from build123d import *

# Parameters (mm, degrees)
ESQUISSE4_R             = 31.794871795
BOSS_EXTRU_1_DEPTH      = 10
ESQUISSE5_R             = 10.8
ESQUISSE5_R_2           = 9
ESQUISSE5_R_3           = 4
BOSS_EXTRU_2_DEPTH      = 10
ESQUISSE6_R             = 4
ENL_V_MAT_EXTRU_2_DEPTH = 5
ESQUISSE8_R             = 4.222540961
ENL_V_MAT_EXTRU_4_DEPTH = 10


with BuildPart() as part:
    # Esquisse4 → Boss.-Extru.1 (new body)
    with BuildSketch(Plane.XY):
        Circle(ESQUISSE4_R)
    extrude(amount=-BOSS_EXTRU_1_DEPTH)

    # Esquisse5 → Boss.-Extru.2 (add)
    # profile 1 of 6: a face of its own
    with BuildSketch(Plane.XY):
        with Locations((15.588457268, -9)):
            Circle(ESQUISSE5_R)
        with Locations((15.588457268, -9)):
            Circle(ESQUISSE5_R_2, mode=Mode.SUBTRACT)
    # profile 2 of 6: a face of its own
    with BuildSketch(Plane.XY):
        with Locations((-15.588457268, -9)):
            Circle(ESQUISSE5_R)
        with Locations((-15.588457268, -9)):
            Circle(ESQUISSE5_R_2, mode=Mode.SUBTRACT)
    # profile 3 of 6: a face of its own
    with BuildSketch(Plane.XY):
        with Locations((0, 18)):
            Circle(ESQUISSE5_R)
        with Locations((0, 18)):
            Circle(ESQUISSE5_R_2, mode=Mode.SUBTRACT)
    # profile 4 of 6: a face of its own
    with BuildSketch(Plane.XY):
        with Locations((21.650635095, 12.5)):
            Circle(ESQUISSE5_R_3)
    # profile 5 of 6: a face of its own
    with BuildSketch(Plane.XY):
        with Locations((-21.650635095, 12.5)):
            Circle(ESQUISSE5_R_3)
    # profile 6 of 6: a face of its own
    with BuildSketch(Plane.XY):
        with Locations((0, -25)):
            Circle(ESQUISSE5_R_3)
    extrude(amount=BOSS_EXTRU_2_DEPTH)

    # Esquisse6 → Enlèv. mat.-Extru.2 (cut)
    with BuildSketch(Plane(origin=(0, 0, -10), x_dir=(-1, 0, 0), z_dir=(0, 0, -1))):
        with Locations((0, 25.641025641)):
            Circle(ESQUISSE6_R)
        with Locations((22.205779584, 12.820512821)):
            Circle(ESQUISSE6_R)
        with Locations((22.205779584, -12.820512821)):
            Circle(ESQUISSE6_R)
        with Locations((0, -25.641025641)):
            Circle(ESQUISSE6_R)
        with Locations((-22.205779584, -12.820512821)):
            Circle(ESQUISSE6_R)
        with Locations((-22.205779584, 12.820512821)):
            Circle(ESQUISSE6_R)
    extrude(amount=-ENL_V_MAT_EXTRU_2_DEPTH, mode=Mode.SUBTRACT)

    # Esquisse8 → Enlèv. mat.-Extru.4 (cut)
    with BuildSketch(Plane(origin=(0, 0, -10), x_dir=(-1, 0, 0), z_dir=(0, 0, -1))):
        Circle(ESQUISSE8_R)
    extrude(amount=-ENL_V_MAT_EXTRU_4_DEPTH, mode=Mode.SUBTRACT)


solid = part.part
Here's how the part is built. I have some questions about the finished solid (model axes, mm). A direction names the side the tool comes from. Coordinates: 2 decimals unless noted, no trailing zeros. Order: outer loops, then holes, each group sorted by start corner. A loop starts at its lowest first (then second) coordinate and runs counter-clockwise, first axis right, second up.
Item 1: If we section it at A-A on x = 0: List the corners of the cut face in (y, z) for me, plus the area to 3 significant figures.
Result sheet:
outline: (-31.79, -10) - (-29.64, -10) - (-29.64, -5) - (-21.64, -5) - (-21.64, -10) - (-4.22, -10) - (-4.22, 0) - (-21, 0) - (-21, 10) - (-29, 10) - (-29, 0) - (-31.79, 0) - close; (4.22, -10) - (21.64, -10) - (21.64, -5) - (29.64, -5) - (29.64, -10) - (31.79, -10) - (31.79, 0) - (28.8, 0) - (28.8, 10) - (27, 10) - (27, 0) - (9, 0) - (9, 10) - (7.2, 10) - (7.2, 0) - (4.22, 0) - close
area: 587 mm2
Item 2: If we mould it in two halves opening along X, with no side actions, what happens to faces 1 (the face through (13, 0, 10)), 2 (the face through (-0.521, -21.034, 4.93)), 3 (the face through (-1.172, 26.923, 4.93))? For each: +X half, -X half, draft (parallel to the pull), parting line (faces both ways), or undercut.
Result sheet:
face 1: draft
face 2: parting line
face 3: undercut
Item 3: If we section it at D-D on y = 23.5: List the corners of the cut face in (x, z) for me.
Result sheet:
outline: (-21.42, -10) - (-3.38, -10) - (-3.38, -5) - (3.38, -5) - (3.38, -10) - (21.42, -10) - (21.42, 0) - (9.29, 0) - (9.29, 10) - (7.12, 10) - (7.12, 0) - (-7.12, 0) - (-7.12, 10) - (-9.29, 10) - (-9.29, 0) - (-21.42, 0) - close
Item 4: For faces 4 (the face through (15, -9, 0)), 5 (the face through (-22, 13, 10)), 6 (the face through (-21.339, -16.725, -7.535)), which set-ups out of +Z, -Z, +X, -X, +Y, -Y let a thin tool reach every point of the face, with its end or its side?
Result sheet:
face 4: +Z
face 5: +Z, +X, -X, +Y, -Y
face 6: -Z
Item 5: If we section it at C-C on z = -1: List the corners of the cut face in (x, y) for me, plus the area to 3 significant figures.
Result sheet:
outline: circle Ø63.59 at (0, 0); hole circle Ø8.45 at (0, 0)
area: 3,120 mm2
Item 6: For P1, Ø6.5, axis at x = 22.21, y = 12.82, coming from the -Z side; P2, Ø1, axis at y = -4.5, z = 5, coming from the -X side; P3, Ø1.5, axis at x = -9.5, z = -2, coming from the +Y side, each with a flat end and sliding along its axis, tell me the tip position at first contact or that it passes through.
Result sheet:
P1: stops at z = -5
P2: stops at x = -25.62
P3: stops at y = 30.57
Item 7: If we section it at B-B on z = 2.25: State how many separate pieces and enclosed holes the cut face has, plus the area to 3 significant figures.
Result sheet:
separate pieces: 6
enclosed holes: 3
area: 487 mm2
Item 8: I need wall thicknesses on line 1 (X direction, y = -15, z = -9); line 2 (X direction, y = 13, z = 7.5); line 3 (Y direction, x = 24.5, z = -6.25). Which ranges of each line are inside material? Lowest first, please.
Result sheet:
line 1: x = -28.03 to -25.56, -18.85 to 18.85, 25.56 to 28.03
line 2: x = -25.62 to -17.68, -9.57 to -7.48, 7.48 to 9.57, 17.68 to 25.62
line 3: y = -20.26 to -16.1, -9.54 to 9.54, 16.1 to 20.26
